```python
from build123d import *

# Parameters (mm, degrees)
F1_DEPTH = 152.4
F2_W     = 101.6
F2_H     = 76.2
F3_DEPTH = 25.4
F4_W     = 76.2
F4_H     = 101.6
F5_DEPTH = 76.2
F7_D     = 6.35
F9_DEPTH = 76.2
F11_D    = 12.7


with BuildPart() as f1:
    # F0 (on Right) → F1 (new body)
    with BuildSketch(Plane.YZ):
        Polygon((0, 100.770188), (-50.8, 100.770188), (-50.8, -102.429812), (101.6, -102.429812), (101.6, -51.629812), (0, -51.629812), align=None)
    extrude(amount=F1_DEPTH)

    # F2 (on face) → F3 (join)
    with BuildSketch(Plane.XY.offset(-51.629812)):
        with Locations((101.6, 63.5)):
            Rectangle(F2_W, F2_H)
        Polygon((152.4, 25.4), (50.8, 25.4), (50.8, 101.6), (0, 101.6), (0, 0), (152.4, 0), align=None)
    extrude(amount=F3_DEPTH)

    # F4 (on face) → F5 (join)
    with BuildSketch(Plane.XY.offset(-26.229812)):
        with Locations((38.1, 50.8)):
            Rectangle(F4_W, F4_H)
    extrude(amount=F5_DEPTH)

    # F7 (through all)
    with Locations(Plane.XY.offset(-26.229812)):
        with Locations((115.396917, 47.733858)):
            Hole(F7_D / 2)

    # F8 (on face) → F9 (cut)
    with BuildSketch(Plane.YZ.offset(76.2)):
        Polygon((101.6, 49.970188), (0, 49.970188), (101.6, -26.229812), align=None)
    extrude(amount=-F9_DEPTH, mode=Mode.SUBTRACT)

    # F11 (through all)
    with Locations(Plane(origin=(0, 0, 0), x_dir=(-1, 0, 0), z_dir=(0, 1, 0))):
        with Locations((-114.3, 63.836917)):
            Hole(F11_D / 2)


solid = f1.part
```
Read the model definition and answer for the solid it produces. Units are mm, in the model's axes. A direction names the side the tool comes from. Give positions to 0.01 mm unless a question says otherwise; leave off trailing zeros. Loops run counter-clockwise (first coordinate to the right, second up) from the corner with the lowest first, then second, coordinate; pieces in that order, holes last.
Item 1: For faces 1 (the flat face through (76.2, 39, 3)), 2 (the flat face through (152.4, -10, -25)), determine the directions among +Z, -Z, +X, -X, +Y, -Y from which every point of the face is accessible in a straight line to the end or side of a thin tool.
Item 2: The part is cut by section B-B (y = 14). Write down the section's boundary in (x, z), and give its area (3 significant figures).
Item 3: The mould has two halves that part along Y. Classify faces 3 (the flat face through (38.633, 50.089, 12.404)), 4 (the cylindrical face through (107.956, -25.756, 64.116)), 5 (the flat face through (75, -50.8, 1)), 6 (the cylindrical face through (112.464, 46.518, -64.863)): released by +Y, released by -Y, zero draft, split by the parting line, or undercut.
Item 4: Each of these flat-tipped pins is pushed along its axis until it touches: pin 1 Ø7.5 at (x, y) = (115.4, 47.73) entering from +Z; pin 2 Ø23 at (y, z) = (45.5, -4) entering from +X; pin 3 Ø10 at (x, z) = (114.3, 63.84) entering from +Y. Where does it stop, or does it pass through?
Item 5: The part is cut by section A-A (x = 95). Write down the section's boundary in (y, z).
Item 6: Find the intervals of material crossed by line 1 along Y through (x, z) = (140, 15); line 2 along Z through (x, y) = (92, 4.5); line 3 along X through (y, z) = (45.5, -71), in increasing order.
Taken from the geometry:
1. face 1: +Z, +X, +Y
1. face 2: +Z, -Z, +X, +Y, -Y
2. outline: (0, -102.43) - (152.4, -102.43) - (152.4, -26.23) - (76.2, -26.23) - (76.2, 39.47) - (0, 39.47) - close
2. area: 16,600 mm2
3. face 3: released by +Y
3. face 4: zero draft
3. face 5: released by -Y
3. face 6: undercut
4. pin 1: stops at z = -26.23
4. pin 2: stops at x = 76.2
4. pin 3: passes through
5. outline: (-50.8, -102.43) - (101.6, -102.43) - (101.6, -26.23) - (0, -26.23) - (0, 100.77) - (-50.8, 100.77) - close
6. line 1: y = -50.8 to 0
6. line 2: z = -102.43 to -26.23
6. line 3: x = 0 to 113.14, 117.65 to 152.4
